```python
from build123d import *

# Parameters (mm, degrees)
CYLINDER003_R     = 1.5
CYLINDER003_DEPTH = 2
CYLINDER001_R     = 5
CYLINDER001_DEPTH = 3
CYLINDER_R        = 6
CYLINDER_DEPTH    = 2
CYLINDER002_R     = 1.5
CYLINDER002_DEPTH = 2


with BuildPart() as cylinder003:
    # Cylinder003 → Cylinder003 (new body)
    with BuildSketch(Plane(origin=(0, 7, 0), x_dir=(1, 0, 0), z_dir=(0, 0, 1))):
        Circle(CYLINDER003_R)
    extrude(amount=CYLINDER003_DEPTH)


with BuildPart() as cylinder001:
    # Cylinder001 → Cylinder001 (new body)
    with BuildSketch(Plane.XY):
        Circle(CYLINDER001_R)
    extrude(amount=CYLINDER001_DEPTH)


with BuildPart() as cut:
    # Cylinder → Cylinder (new body)
    with BuildSketch(Plane.XY):
        Circle(CYLINDER_R)
    extrude(amount=CYLINDER_DEPTH)

    # Cut: cut Cylinder001
    add(cylinder001.part, mode=Mode.SUBTRACT)


with BuildPart() as fusion:
    # Cylinder002 → Cylinder002 (new body)
    with BuildSketch(Plane(origin=(-7, 0, 0), x_dir=(1, 0, 0), z_dir=(0, 0, 1))):
        Circle(CYLINDER002_R)
    extrude(amount=CYLINDER002_DEPTH)

    # Fusion: union Cylinder003, Cut
    add(cylinder003.part)
    add(cut.part)


solid = fusion.part
```
Could you check a few things on this model? Use its own coordinates, in mm. Round coordinates to 2 decimals unless told otherwise and drop trailing zeros. Write each loop counter-clockwise with the first axis right and the second up, starting at its lowest first coordinate (ties: lowest second). Pieces come first, ordered by that corner, then holes. Notation, with made-up numbers: M -29,18.25 L 27,18.25 A4 cw 27,24.25 Z; hole C 8,-34.5 d6. An arc over 180 degrees is marked long. Answer in a Markdown table with one row per item. Add a question column.
Q1. Imagine slicing it at C-C (z = 1.8). Please give me the cut outline in (x, y), then the cut area to 3 significant figures.
Q2. If we mould it in two halves opening along Y, with no side actions, what happens to faces 1 (the cylindrical face through (-1.08, -4.88, 0.99)), 2 (the flat face through (-5, 2, 0))? For each: +Y half, -Y half, draft (parallel to the pull), parting line (faces both ways), or undercut.
Q3. If I drill on line 1 (X direction, y = 0, z = 1.1); line 2 (Y direction, x = 0, z = 1.15); line 3 (X direction, y = -2.5, z = 1.1), over which ranges is the centre line in solid material (lowest first)? Write a range as from..to.
Q4. Imagine slicing it at A-A (y = 0). Please give me the cut outline in (x, z).
Q5. Imagine slicing it at B-B (x = 0). Please give me the cut outline in (y, z).
Q6. Imagine slicing it at D-D (x = -7). Please give me the cut outline in (y, z), then the cut area to 3 significant figures.
Values:
| question | item | result |
|---|---|---|
| 1 | outline | M -5.91,-1.03 A6 ccw long 1.03,5.91 A1.5 ccw long -1.03,5.91 A6 ccw -5.91,1.03 A1.5 ccw long Z; hole C 0,0 d10 |
| 1 | area | 47.3 mm^2 |
| 2 | face 1 | undercut |
| 2 | face 2 | draft |
| 3 | line 1 | -8.5..-5, 5..6 |
| 3 | line 2 | -6..-5, 5..8.5 |
| 3 | line 3 | -5.45..-4.33, 4.33..5.45 |
| 4 | outline | M -8.5,0 L -5,0 L -5,2 L -8.5,2 Z; M 5,0 L 6,0 L 6,2 L 5,2 Z |
| 5 | outline | M -6,0 L -5,0 L -5,2 L -6,2 Z; M 5,0 L 8.5,0 L 8.5,2 L 5,2 Z |
| 6 | outline | M -1.5,0 L 1.5,0 L 1.5,2 L -1.5,2 Z |
| 6 | area | 6.00 mm^2 |
